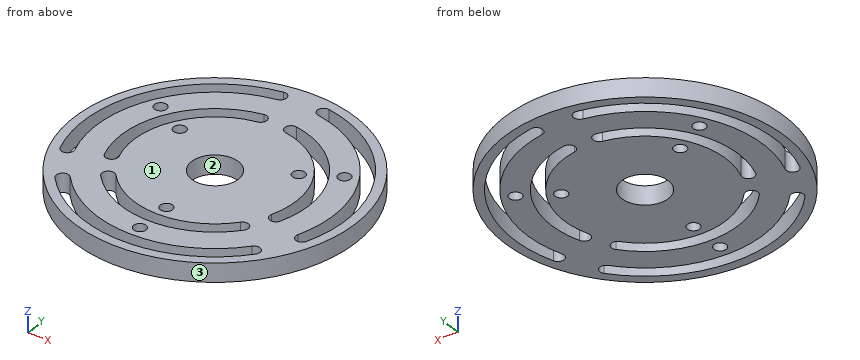
Autodesk Inventor part; units mm, degrees
ref_plane "YZ Plane" through (0, 0, 0) normal (1, 0, 0) x (0, 1, 0)
ref_plane "XZ Plane" through (0, 0, 0) normal (0, 1, 0) x (-1, 0, 0)
ref_plane "XY Plane" through (0, 0, 0) normal (0, 0, 1) x (1, 0, 0)
sketch "Sketch1" plane through (0, 0, 0) normal (0, 0, 1) x (1, 0, 0)
  line L0 (0, 63) -> (0, -63)
  line L1 (-63, 0) -> (63, 0)
  circle A0 centre (0, 0) radius 45
  dimension "d0" = 90
extrude "Extrusion1" add sketch "Sketch1" along normal blind 6
sketch "Sketch2" plane through (0, 0, 6) normal (0, 0, 1) x (1, 0, 0)
  circle A0 centre (0, 0) radius 7.5
  circle A1 centre (0, 0) radius 45
  line L0 (0, 63) -> (0, -63)
  line L1 (-63, 0) -> (63, 0)
  arc A2 (-21.4492, -17.9981) -> (21.4492, -17.9981) centre (0, 0) ccw construction
  arc A3 (-22.9813, -19.2836) -> (22.9813, -19.2836) centre (0, 0) ccw
  arc A4 (-19.9172, -16.7125) -> (19.9172, -16.7125) centre (0, 0) ccw
  arc A5 (-19.9172, -16.7125) -> (-22.9813, -19.2836) centre (-21.4492, -17.9981) ccw
  arc A6 (22.9813, -19.2836) -> (19.9172, -16.7125) centre (21.4492, -17.9981) ccw
  line L2 (0, 0) -> (21.4492, -17.9981) construction
  line L3 (0, 0) -> (-21.4492, -17.9981) construction
  arc A7 (-30.6418, -25.7115) -> (30.6418, -25.7115) centre (0, 0) ccw construction
  arc A8 (-32.1739, -26.9971) -> (32.1739, -26.9971) centre (0, 0) ccw
  arc A9 (-29.1097, -24.4259) -> (29.1097, -24.4259) centre (0, 0) ccw
  arc A10 (-29.1097, -24.4259) -> (-32.1739, -26.9971) centre (-30.6418, -25.7115) ccw
  arc A11 (32.1739, -26.9971) -> (29.1097, -24.4259) centre (30.6418, -25.7115) ccw
  line L4 (0, 0) -> (30.6418, -25.7115) construction
  line L5 (0, 0) -> (-30.6418, -25.7115) construction
  circle A12 centre (0, -34) radius 2
  circle A13 centre (0, -22) radius 2
  dimension "d3" = 15
  dimension "d35" = 100
  dimension "d36" = 4
  dimension "d37" = 28
  dimension "d38" = 100
  dimension "d39" = 4
  dimension "d40" = 12
  dimension "d41" = 4
  dimension "d42" = 4
  dimension "d43" = 22
  dimension "d44" = 34
extrude "Extrusion2" cut sketch "Sketch2" against normal through all contours L1 L0 A0 | A0 L0 L1 | L0 L1 A0 | A0 L1 L0 | A13 L0 | L0 A13 | A8 A10 A9 L0 | L0 A9 A11 A8 | A4 A6 A3 L0 | L0 A3 A5 A4 | A12 L0 | L0 A12
pattern_circular "Circular Pattern2" count 3 over 360 about axis through (0, 0, 6) along (0, 0, -1) of "Extrusion2"
properties part number "WorkTriangleDisk"
Work out the finished part from the listing and answer in its coordinate system (mm). Face numbers are marked on the shaded views. Coordinates: 2 decimals unless noted, no trailing zeros. Write each loop counter-clockwise with the first axis right and the second up, starting at its lowest first coordinate (ties: lowest second). Pieces come first, ordered by that corner, then holes.
1. The part is cut by section D-D, the plane y = -34. Write down the section's boundary in (x, z).
Results list:
outline: (-29.48, 0) - (-24.66, 0) - (-24.66, 6) - (-29.48, 6) - close; (-16.97, 0) - (-2, 0) - (-2, 6) - (-16.97, 6) - close; (2, 0) - (16.97, 0) - (16.97, 6) - (2, 6) - close; (24.66, 0) - (29.48, 0) - (29.48, 6) - (24.66, 6) - close
2. The part is cut by section B-B, the plane x = 0. Write down the section's boundary in (y, z), and give its area (3 significant figures).
Results list:
outline: (-45, 0) - (-42, 0) - (-42, 6) - (-45, 6) - close; (-38, 0) - (-36, 0) - (-36, 6) - (-38, 6) - close; (-32, 0) - (-30, 0) - (-30, 6) - (-32, 6) - close; (-26, 0) - (-24, 0) - (-24, 6) - (-26, 6) - close; (-20, 0) - (-7.5, 0) - (-7.5, 6) - (-20, 6) - close; (7.5, 0) - (45, 0) - (45, 6) - (7.5, 6) - close
area: 354 mm2
3. Flat-ended cylindrical pins translate along their axes: pin 1 (2 mm diameter, centred on x = 19, y = -3.5, fed in from -Z); pin 2 (13.5 mm diameter, centred on x = 0, y = 0, fed in from -Z). Find the tip coordinate at first contact, or state that the pin passes through.
Results list:
pin 1: stops at z = 0
pin 2: passes through
4. The part is cut by section C-C, the plane z = 4.1. State how many separate pieces and enclosed holes the cut face has, and give its area (3 significant figures).
Results list:
separate pieces: 1
enclosed holes: 13
area: 4,610 mm2
5. The part is cut by section A-A, the plane y = 0. Write down the section's boundary in (x, z).
Results list:
outline: (-45, 0) - (-42, 0) - (-42, 6) - (-45, 6) - close; (-38, 0) - (-30, 0) - (-30, 6) - (-38, 6) - close; (-26, 0) - (-7.5, 0) - (-7.5, 6) - (-26, 6) - close; (7.5, 0) - (26, 0) - (26, 6) - (7.5, 6) - close; (30, 0) - (38, 0) - (38, 6) - (30, 6) - close; (42, 0) - (45, 0) - (45, 6) - (42, 6) - close
6. Consider line 1 along Y through (x, z) = (0, 3.15); line 2 along X through (y, z) = (0, 3.75); line 3 along X through (y, z) = (31, 2.35). Determine where each line is inside the solid, lowest interval first.
Results list:
line 1: y = -45 to -42, -38 to -36, -32 to -30, -26 to -24, -20 to -7.5, 7.5 to 45
line 2: x = -45 to -42, -38 to -30, -26 to -7.5, 7.5 to 26, 30 to 38, 42 to 45
line 3: x = -32.62 to -28.34, -21.98 to 21.98, 28.34 to 32.62
7. For a pull along Y with two mould halves and no side action, classify the marked faces 1, 2 and 3 as +Y half, -Y half, draft (parallel to the pull), parting line (faces both ways), or undercut.
Results list:
face 1: draft
face 2: undercut
face 3: parting line
